Can you work these out from the model? Positions are in its coordinate system, mm. Face numbers are marked on the shaded views. Coordinates: 2 decimals unless noted, no trailing zeros. Order: outer loops, then holes, each group sorted by start corner. A loop starts at its lowest first (then second) coordinate and runs counter-clockwise, first axis right, second up. Notation, with made-up numbers: M -27,82 L 2,82 A22 cw 2,118 Z; hole C 52.25,-37 d10. An arc over 180 degrees is marked long. Answer as a JSON object with one key per item and string values.
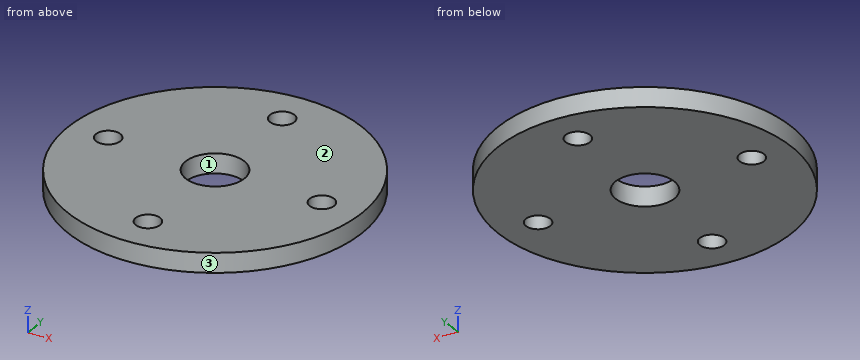
from build123d import *

# Parameters (mm, degrees)
ESQUISSE1_R        = 75
ESQUISSE1_R_2      = 15
ESQUISSE1_R_3      = 6.25
BOSS_EXTRU_1_DEPTH = 5


with BuildPart() as part:
    # Esquisse1 → Boss.-Extru.1 (new body, symmetric)
    with BuildSketch(Plane.XY):
        Circle(ESQUISSE1_R)
        Circle(ESQUISSE1_R_2, mode=Mode.SUBTRACT)
        with Locations((0, 55)):
            Circle(ESQUISSE1_R_3, mode=Mode.SUBTRACT)
        with Locations((-55, 0)):
            Circle(ESQUISSE1_R_3, mode=Mode.SUBTRACT)
        with Locations((0, -55)):
            Circle(ESQUISSE1_R_3, mode=Mode.SUBTRACT)
        with Locations((55, 0)):
            Circle(ESQUISSE1_R_3, mode=Mode.SUBTRACT)
    extrude(amount=BOSS_EXTRU_1_DEPTH, both=True)


solid = part.part
Item 1: Please list where these lines run through material, in increasing order: line 1 (Y direction, x = 0, z = 2.75); line 2 (Y direction, x = -55, z = 0); line 3 (X direction, y = -12, z = -0.75).
Answers follow:
{"line 1": "y = -75 to -61.25, -48.75 to -15, 15 to 48.75, 61.25 to 75", "line 2": "y = -50.99 to -6.25, 6.25 to 50.99", "line 3": "x = -74.03 to -9, 9 to 74.03"}
Item 2: If we mould it in two halves opening along X, with no side actions, what happens to the marked faces 1, 2 and 3? For each: pulls with the +X half, pulls with the -X half, needs draft (parallel to the pull), parting line crosses it, or undercut.
Answers follow:
{"face 1": "undercut", "face 2": "needs draft", "face 3": "parting line crosses it"}
Item 3: I want a section at D-D, the plane x = 55. Write out the boundary of the cut face in (y, z), plus the area to 3 significant figures.
Answers follow:
{"outline": "M -50.99,-5 L -6.25,-5 L -6.25,5 L -50.99,5 Z; M 6.25,-5 L 50.99,-5 L 50.99,5 L 6.25,5 Z", "area": "895 mm^2"}
Item 4: I want a section at C-C, the plane z = -1.25. Write out the boundary of the cut face in (x, y).
Answers follow:
{"outline": "C 0,0 d150; hole C -55,0 d12.5; hole C 0,0 d30; hole C 0,-55 d12.5; hole C 0,55 d12.5; hole C 55,0 d12.5"}
Item 5: I want a section at A-A, the plane x = 0. Write out the boundary of the cut face in (y, z), plus the area to 3 significant figures.
Answers follow:
{"outline": "M -75,-5 L -61.25,-5 L -61.25,5 L -75,5 Z; M -48.75,-5 L -15,-5 L -15,5 L -48.75,5 Z; M 15,-5 L 48.75,-5 L 48.75,5 L 15,5 Z; M 61.25,-5 L 75,-5 L 75,5 L 61.25,5 Z", "area": "950 mm^2"}
Item 6: I'm going to push flat-ended pins straight in: pin 1 (1 mm diameter, centred on x = -49, z = 1, fed in from +Y); pin 2 (5 mm diameter, centred on y = -17, z = -2.5, fed in from -X) (3 decimals); pin 3 (10 mm diameter, centred on x = 0, y = -55, fed in from +Z); pin 4 (1 mm diameter, centred on y = 31.5, z = 3, fed in from -X). Where does each tip first touch, or does it pass through?
Answers follow:
{"pin 1": "stops at y = 57.21", "pin 2": "stops at x = -73.585", "pin 3": "passes through", "pin 4": "stops at x = -68.29"}
